Here's the drawing with two shaded views (mm, measured from the low corner). I have some questions. Coordinates: 2 decimals unless noted, no trailing zeros. Write each loop counter-clockwise with the first axis right and the second up, starting at its lowest first coordinate (ties: lowest second). Pieces come first, ordered by that corner, then holes.
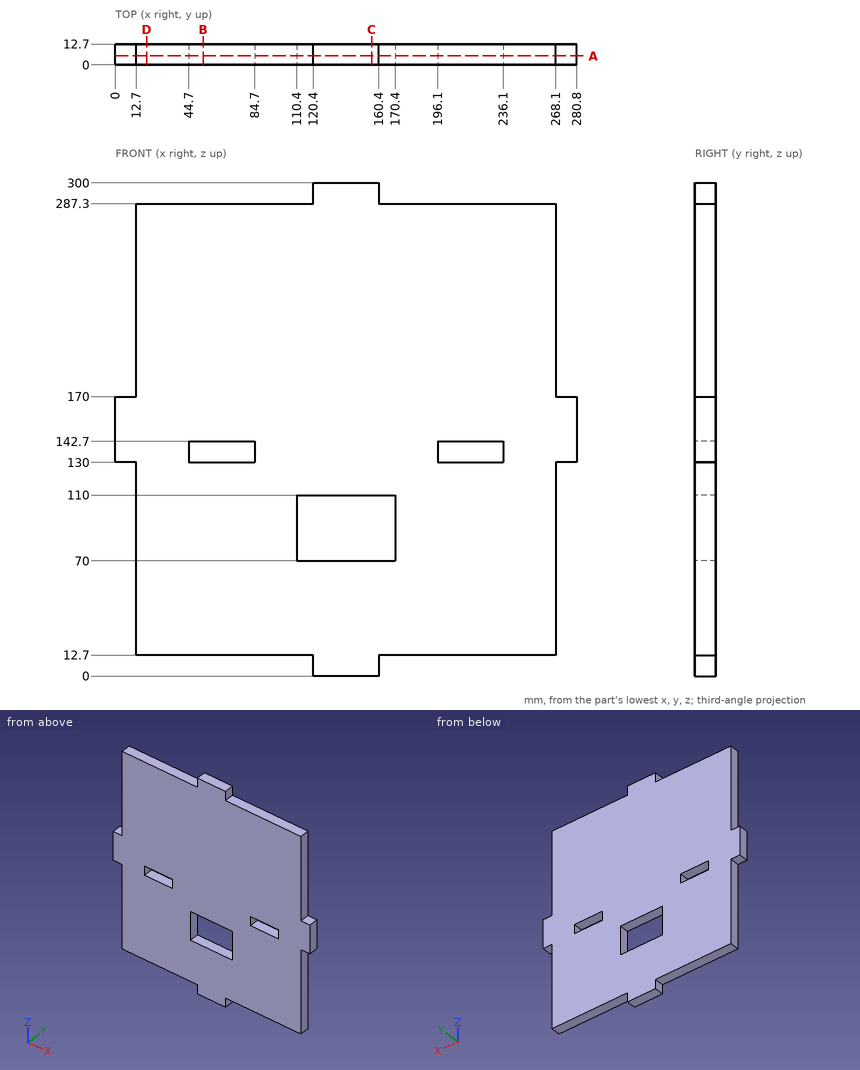
1. I want a section at D-D on x = 19. Please give me the cut outline in (y, z), plus the area to 3 significant figures.
Verdict:
outline: (0, 12.7) - (12.7, 12.7) - (12.7, 287.3) - (0, 287.3) - close
area: 3,490 mm2
2. Please list where these lines run through material, in increasing order: line 1 along Z through (x, y) = (112.5, 10.25); line 2 along Z through (x, y) = (221, 1); line 3 along X through (y, z) = (1, 69).
Verdict:
line 1: z = 12.7 to 70, 110 to 287.3
line 2: z = 12.7 to 130, 142.7 to 287.3
line 3: x = 12.7 to 268.1
3. I want a section at A-A on y = 5.5. Give the number of separate pieces and of enclosed holes in the cut face, plus the area to 3 significant figures.
Verdict:
separate pieces: 1
enclosed holes: 3
area: 68,700 mm2
4. I want a section at B-B on x = 53.5. Please give me the cut outline in (y, z).
Verdict:
outline: (0, 12.7) - (12.7, 12.7) - (12.7, 130) - (0, 130) - close; (0, 142.7) - (12.7, 142.7) - (12.7, 287.3) - (0, 287.3) - close
5. For pin 1 (4 mm diameter, centred on x = 274, y = 4, fed in from +Z); pin 2 (4 mm diameter, centred on y = 5.5, z = 292.5, fed in from -X); pin 3 (6.5 mm diameter, centred on y = 4.5, z = 83, fed in from -X), each with a flat end and sliding along its axis, tell me the tip position at first contact or that it passes through.
Verdict:
pin 1: stops at z = 170
pin 2: stops at x = 120.4
pin 3: stops at x = 12.7
6. I want a section at C-C on x = 156. Please give me the cut outline in (y, z).
Verdict:
outline: (0, 0) - (12.7, 0) - (12.7, 70) - (0, 70) - close; (0, 110) - (12.7, 110) - (12.7, 300) - (0, 300) - close
